Autodesk Inventor part; units mm, degrees
ref_plane "YZ Plane" through (0, 0, 0) normal (1, 0, 0) x (0, 1, 0)
ref_plane "XZ Plane" through (0, 0, 0) normal (0, 1, 0) x (-1, 0, 0)
ref_plane "XY Plane" through (0, 0, 0) normal (0, 0, 1) x (1, 0, 0)
sketch "Sketch1" plane through (0, 0, 0) normal (1, 0, 0) x (0, 1, 0)
  circle A0 centre (0, 0) radius 3
  dimension "d0" = 6
extrude "Extrusion1" add sketch "Sketch1" along normal mid plane 29.5
sketch "Sketch2" plane through (14.75, 0, 0) normal (1, 0, 0) x (0, 0, -1)
  circle A0 centre (0, 0) radius 2.25
  circle A1 centre (0, 0) radius 1.5
  circle A2 centre (0, 0) radius 3
  dimension "d3" = 4.5
  dimension "d4" = 3
extrude "Extrusion2" cut sketch "Sketch2" against normal blind 4.75
sketch "Sketch3" plane through (-14.75, 0, 0) normal (-1, 0, 0) x (0, 0, 1)
  circle A0 centre (0, 0) radius 2.25
  circle A1 centre (0, 0) radius 1.5
  circle A2 centre (0, 0) radius 3
  dimension "d7" = 4.5
  dimension "d8" = 3
  dimension "d9" = 6
extrude "Extrusion3" cut sketch "Sketch3" against normal blind 4.75
sketch "Sketch4" plane through (0, 0, 0) normal (1, 0, 0) x (0, 1, 0)
  circle A0 centre (0, 0) radius 3
  line L0 (3, 0) -> (1.5, 0)
  line L1 (1.5, 3.5) -> (3, 3.5)
  line L2 (3, 3.5) -> (3, -3.5)
  line L3 (3, -3.5) -> (1.5, -3.5)
  line L4 (1.5, -3.5) -> (1.5, 3.5)
  circle A1 centre (0, 0) radius 2.25
  line L5 (1.5, 3.5) -> (3, -3.5) construction
  line L6 (3, 3.5) -> (1.5, -3.5) construction
  point P0 (2.25, 0)
  dimension "d12" = 1.5
  dimension "d13" = 7
extrude "Extrusion4" cut sketch "Sketch4" along normal mid plane 10 contours L0 A1 L4 A0 | L2 L3 L4 A0 | A0 L4 A1 L0 | A0 L4 L1 L2 | A1 L4 L0 | L0 L4 A1
sketch "Sketch5" plane through (-5, 1.5, -2.5981) normal (0, 1, 0) x (1, 0, 0)
  circle A0 centre (5, -2.5981) radius 1.5
  dimension "d16" = 3
extrude "Extrusion5" cut sketch "Sketch5" against normal through all
thread "Thread1"
thread "Thread2"
sketch "Sketch6" plane through (10, 0, 0) normal (1, 0, 0) x (0, 0, -1)
  circle A0 centre (0, 0) radius 1.5
extrude "Extrusion6" cut sketch "Sketch6" against normal blind 2
sketch "Sketch7" plane through (-10, 0, 0) normal (-1, 0, 0) x (0, 0, 1)
  circle A0 centre (0, 0) radius 1.5
extrude "Extrusion7" cut sketch "Sketch7" against normal blind 2
properties part number "Z25_Spacer" material "Aluminum 6061"
The listing builds one solid part. Answer for the finished solid, in the listing's coordinates (mm). A direction names the side the tool comes from. Coordinates: 2 decimals unless noted, no trailing zeros. Order: outer loops, then holes, each group sorted by start corner. A loop starts at its lowest first (then second) coordinate and runs counter-clockwise, first axis right, second up.
Q1. Which of the six approach directions +Z, -Z, +X, -X, +Y, -Y give full straight-line access (tool end or side, diameter ignored) to faces 1 (the face through (-14.75, -2, 0)), 2 (the face through (-5, 2, 0)), 3 (the face through (-8, 0, 0)), 4 (the face through (12.41, 2.23, 0.29))?
Q2. A cutting plane is placed at A-A, the plane z = 0. Write down the section's boundary in (x, y), and give its area (4 significant figures).
Q3. Given P1, Ø1, axis at x = 1.5, z = 0, coming from the +Y side; P2, Ø1, axis at x = -3.5, z = 2.5, coming from the -Y side; P3, Ø0.9, axis at y = 0, z = 0, coming from the -X side, each flat-ended and moving along its own axis, determine where each tip first touches the part or whether it passes through.
Q4. Consider line 1 (X direction, y = -2.5, z = 0); line 2 (Y direction, x = -11, z = 0); line 3 (X direction, y = 1.25, z = 0). Determine where each line is inside the solid, lowest interval first.
Q5. A cutting plane is placed at D-D, the plane x = 9.75. Write down the section's boundary in (y, z).
Q6. A cutting plane is placed at B-B, the plane y = 0. Write down the section's boundary in (x, z), and give its area (3 significant figures).
Q7. For a pull along Y with two mould halves and no side action, classify faces 5 (the face through (5, 2, 0)), 6 (the face through (-11.42, 0.07, -1.5)), 7 (the face through (-0.1, -2.4, 1.8)) as pulls with the +Y half, pulls with the -Y half, needs draft (parallel to the pull), parting line crosses it, or undercut.
Q8. A cutting plane is placed at C-C, the plane x = 0. Write down the section's boundary in (y, z).
Answers follow:
1. face 1: +Z, -Z, -X, +Y, -Y
1. face 2: +Z, -Z, +Y
1. face 3: -X
1. face 4: +X
2. outline: (-14.75, -2.25) - (-10, -2.25) - (-10, -3) - (-1.5, -3) - (-1.5, 1.5) - (-5, 1.5) - (-5, 3) - (-10, 3) - (-10, 2.25) - (-14.75, 2.25) - (-14.75, 1.5) - (-8, 1.5) - (-8, -1.5) - (-14.75, -1.5) - close; (1.5, -3) - (10, -3) - (10, -2.25) - (14.75, -2.25) - (14.75, -1.5) - (8, -1.5) - (8, 1.5) - (14.75, 1.5) - (14.75, 2.25) - (10, 2.25) - (10, 3) - (5, 3) - (5, 1.5) - (1.5, 1.5) - close
2. area: 93.75 mm2
3. P1: stops at y = 1.5
3. P2: stops at y = -2.24
3. P3: stops at x = -8
4. line 1: x = -10 to -1.5, 1.5 to 10
4. line 2: y = -2.25 to -1.5, 1.5 to 2.25
4. line 3: x = -8 to -1.5, 1.5 to 8
5. outline: circle Ø6 at (0, 0); hole circle Ø3 at (0, 0)
6. outline: (-14.75, -2.25) - (-10, -2.25) - (-10, -3) - (10, -3) - (10, -2.25) - (14.75, -2.25) - (14.75, -1.5) - (8, -1.5) - (8, 1.5) - (14.75, 1.5) - (14.75, 2.25) - (10, 2.25) - (10, 3) - (-10, 3) - (-10, 2.25) - (-14.75, 2.25) - (-14.75, 1.5) - (-8, 1.5) - (-8, -1.5) - (-14.75, -1.5) - close; hole circle Ø3 at (0, 0)
6. area: 115 mm2
7. face 5: needs draft
7. face 6: undercut
7. face 7: parting line crosses it
8. outline: (-2.6, -1.5) arc R3 ccw to (1.5, -2.6) - (1.5, -1.5) - close; (-2.6, 1.5) - (1.5, 1.5) - (1.5, 2.6) arc R3 ccw to start
